Work out the finished part from the listing and answer in its coordinate system (mm). A direction names the side the tool comes from. Round coordinates to 2 decimals unless told otherwise and drop trailing zeros. Loops run counter-clockwise (first coordinate to the right, second up) from the corner with the lowest first, then second, coordinate; pieces in that order, holes last.
```python
from build123d import *

# Parameters (mm, degrees)
EXTRUDE_THIN1_DEPTH = 381
FILLET1_R           = 1.27


with BuildPart() as part:
    # Sketch1 → Extrude-Thin1 (new body)
    with BuildSketch(Plane.XY):
        with BuildLine():
            Line((0, 0), (-3.96875, 0))
            ThreePointArc((-3.96875, 0), (-4.818127422, 5.384319506), (-8.48088981, 9.421213144))
            ThreePointArc((-8.48088981, 9.421213144), (-11.680182616, 12.112043916), (-13.902370802, 15.652937077))
            ThreePointArc((-13.902370802, 15.652937077), (-13.70628274, 19.809085553), (-10.31875, 22.225))
            Line((-10.31875, 22.225), (-10.31875, 25.4))
            Line((-10.31875, 25.4), (23.8125, 25.4))
            Line((23.8125, 25.4), (23.8125, 24.13))
            Line((23.8125, 24.13), (-9.04875, 24.13))
            Line((-9.04875, 24.13), (-9.04875, 20.988987709))
            ThreePointArc((-9.04875, 20.988987709), (-12.302505111, 19.646426389), (-12.735071921, 16.153250302))
            ThreePointArc((-12.735071921, 16.153250302), (-10.722030859, 12.945617675), (-7.823847964, 10.508041563))
            ThreePointArc((-7.823847964, 10.508041563), (-4.006030041, 6.572994806), (-2.613703655, 1.27))
            Line((-2.613703655, 1.27), (0, 1.27))
            Line((0, 1.27), (0, 0))
        make_face()
    extrude(amount=-EXTRUDE_THIN1_DEPTH)

    # Fillet1
    fillet1_edges = [part.edges().sort_by_distance(p)[0] for p in [
        (-9.04875, 20.988987709, -190.5),
        (-3.96875, 0, -190.5),
        (-10.31875, 25.4, -190.5),
    ]]
    fillet(fillet1_edges, radius=FILLET1_R)


solid = part.part
```
1. Find section B-B (x = 18). Write down the section's boundary in (y, z).
Answer key:
outline: (24.13, -381) - (25.4, -381) - (25.4, 0) - (24.13, 0) - close
2. Which of the six approach directions +Z, -Z, +X, -X, +Y, -Y give full straight-line access (tool end or side, diameter ignored) to faces 1 (the face through (-11.642, 12.068, -187.833)), 2 (the face through (8, 24.13, -188))?
Answer key:
face 1: +Z, -Z, -X, -Y
face 2: +Z, -Z, +X
3. Given pin 1 (1 mm diameter, centred on y = 1, z = -105, fed in from +X); pin 2 (1.5 mm diameter, centred on y = 20, z = -178, fed in from -X); pin 3 (1 mm diameter, centred on y = 23, z = -203, fed in from -X), each flat-ended and moving along its own axis, determine where each tip first touches the part or whether it passes through.
Answer key:
pin 1: stops at x = 0
pin 2: stops at x = -13.97
pin 3: stops at x = -10.32
4. Consider probe 1 along X at (y, z) = (24, -277); probe 2 along Y at (x, z) = (-10, -255); probe 3 along Y at (x, z) = (7.5, -209.5). Determine where each line is inside the solid, lowest interval first.
Answer key:
probe 1: x = -10.32 to -9.05
probe 2: y = 10.49 to 12.18, 21 to 24.97
probe 3: y = 24.13 to 25.4
